CAD build for the part. Positions are in the model's coordinates, mm. A direction names the side the tool comes from. Give positions to 0.01 mm unless a question says otherwise; leave off trailing zeros. Write each loop counter-clockwise with the first axis right and the second up, starting at its lowest first coordinate (ties: lowest second). Pieces come first, ordered by that corner, then holes. Notation, with made-up numbers: (-21.5, 17.5) - (-7.5, 17.5) arc R24 cw to (-7.5, 34.5) - close; hole circle Ø6 at (1.25, 85). An arc over 180 degrees is marked (long way). Put each result on its own line as item: value. Start each with the question number.
1. Tool access for faces 1 (the cylindrical face through (-11.273, 178.043, -387.92)), 2 (the cylindrical face through (9.113, 196.684, -489.814)), 3 (the flat face through (-21, 47, 5)): list every direction of +Z, -Z, +X, -X, +Y, -Y with a clear straight run to the whole face (end or side of a thin tool).
2. Wall check: line 1 (Y direction, x = 30, z = -488); line 2 (Z direction, x = -25, y = 78); line 3 (X direction, y = -36, z = -171). Give the ranges that are in metal, low to high.
3. Cut at B-B on z = -130. List the corners of the cut face in (x, y).
4. Cut at C-C on x = -16.5. List the corners of the cut face in (y, z), and give its area (3 significant figures).
5. Cut at A-A on x = -44. List the corners of the cut face in (y, z).
6. Mould opens along X. For faces 4 (the flat face through (52, 122, -487.279)), 5 (the cylindrical face through (-49.95, 63.18, -246.29)), 6 (the cylindrical face through (-55.55, -42.594, 2.465)) say: +X half, -X half, draft (parallel to the pull), parting line (faces both ways), or undercut.
7. Drop flat-ended pins along their axis: pin 1 (5 mm diameter, centred on x = -11.5, y = 119.5, fed in from +Z); pin 2 (4.5 mm diameter, centred on x = 0, y = -60, fed in from +Z); pin 3 (4.5 mm diameter, centred on x = -30, y = 51.96, fed in from +Z); pin 4 (10 mm diameter, centred on x = 40, y = -33.5, fed in from -Z). Give the stop position or say it passes through.
from build123d import *

# Parameters (mm, degrees)
SKETCH2_R           = 52
SKETCH2_R_2         = 50
SKETCH4_R           = 70
SKETCH4_R_2         = 50
SKETCH4_R_3         = 2.5
BOSS_EXTRUDE1_DEPTH = 5
BOSS_EXTRUDE2_START = 5
SKETCH5_R           = 70
SKETCH5_R_2         = 50
SKETCH5_R_3         = 2.5
BOSS_EXTRUDE2_DEPTH = 5


with BuildPart() as part:
    # Sweep-Thin1: sweep along a path in Sketch3
    with BuildLine(Plane(origin=(0, 0, 0), x_dir=(0, 0, -1), z_dir=(1, 0, 0))) as sweep_thin1_path:
        Line((0, 0), (180, 0))
        Line((180, 0), (307.279220614, 127.279220614))
        Line((307.279220614, 127.279220614), (487.279220614, 127.279220614))
    # Sketch2 → Sweep-Thin1 (sweep)
    with BuildSketch(Plane.XY):
        Circle(SKETCH2_R)
        Circle(SKETCH2_R_2, mode=Mode.SUBTRACT)
    sweep(path=sweep_thin1_path.line, transition=Transition.RIGHT)

    # Sketch4 → Boss-Extrude1 (add)
    with BuildSketch(Plane.XY):
        Circle(SKETCH4_R)
        with Locations(Location((0, 0, 0), (0, 0, 90))):
            Circle(SKETCH4_R_2, mode=Mode.SUBTRACT)
        with Locations((0, -60)):
            Circle(SKETCH4_R_3, mode=Mode.SUBTRACT)
        with Locations((-30, -51.961524227)):
            Circle(SKETCH4_R_3, mode=Mode.SUBTRACT)
        with Locations((-51.961524227, -30)):
            Circle(SKETCH4_R_3, mode=Mode.SUBTRACT)
        with Locations((-60, 0)):
            Circle(SKETCH4_R_3, mode=Mode.SUBTRACT)
        with Locations((-51.961524227, 30)):
            Circle(SKETCH4_R_3, mode=Mode.SUBTRACT)
        with Locations((-30, 51.961524227)):
            Circle(SKETCH4_R_3, mode=Mode.SUBTRACT)
        with Locations((0, 60)):
            Circle(SKETCH4_R_3, mode=Mode.SUBTRACT)
        with Locations((30, 51.961524227)):
            Circle(SKETCH4_R_3, mode=Mode.SUBTRACT)
        with Locations((51.961524227, 30)):
            Circle(SKETCH4_R_3, mode=Mode.SUBTRACT)
        with Locations((60, 0)):
            Circle(SKETCH4_R_3, mode=Mode.SUBTRACT)
        with Locations((51.961524227, -30)):
            Circle(SKETCH4_R_3, mode=Mode.SUBTRACT)
        with Locations((30, -51.961524227)):
            Circle(SKETCH4_R_3, mode=Mode.SUBTRACT)
    extrude(amount=BOSS_EXTRUDE1_DEPTH)

    # Sketch5 → Boss-Extrude2 (add)
    with BuildSketch(Plane(origin=(0, 0, -487.279220614), x_dir=(-1, 0, 0), z_dir=(0, 0, -1)).offset(BOSS_EXTRUDE2_START)):
        with Locations((0, 127.279220614)):
            Circle(SKETCH5_R)
        with Locations((0, 127.279220614)):
            Circle(SKETCH5_R_2, mode=Mode.SUBTRACT)
        with Locations((0, 67.279220614)):
            Circle(SKETCH5_R_3, mode=Mode.SUBTRACT)
        with Locations((-30, 75.317696387)):
            Circle(SKETCH5_R_3, mode=Mode.SUBTRACT)
        with Locations((-51.961524227, 97.279220614)):
            Circle(SKETCH5_R_3, mode=Mode.SUBTRACT)
        with Locations((-60, 127.279220614)):
            Circle(SKETCH5_R_3, mode=Mode.SUBTRACT)
        with Locations((-51.961524227, 157.279220614)):
            Circle(SKETCH5_R_3, mode=Mode.SUBTRACT)
        with Locations((-30, 179.240744841)):
            Circle(SKETCH5_R_3, mode=Mode.SUBTRACT)
        with Locations((0, 187.279220614)):
            Circle(SKETCH5_R_3, mode=Mode.SUBTRACT)
        with Locations((30, 179.240744841)):
            Circle(SKETCH5_R_3, mode=Mode.SUBTRACT)
        with Locations((51.961524227, 157.279220614)):
            Circle(SKETCH5_R_3, mode=Mode.SUBTRACT)
        with Locations((60, 127.279220614)):
            Circle(SKETCH5_R_3, mode=Mode.SUBTRACT)
        with Locations((51.961524227, 97.279220614)):
            Circle(SKETCH5_R_3, mode=Mode.SUBTRACT)
        with Locations((30, 75.317696387)):
            Circle(SKETCH5_R_3, mode=Mode.SUBTRACT)
    extrude(amount=-BOSS_EXTRUDE2_DEPTH)


solid = part.part
Report:
1. face 1: none
1. face 2: -Z
1. face 3: +Z, +X, -X, +Y, -Y
2. line 1: y = 64.03 to 72.82, 77.82 to 87.28, 167.28 to 176.74, 181.74 to 190.52
2. line 2: z = -492.28 to -487.28, -322.48 to -319.24, -196.76 to -193.52
2. line 3: x = -37.52 to -34.7, 34.7 to 37.52
3. outline: circle Ø104 at (0, 0); hole circle Ø100 at (0, 0)
4. outline: (-68.03, 0) - (-49.31, 0) - (-49.31, -200.43) - (77.97, -327.71) - (77.97, -487.28) - (59.25, -487.28) - (59.25, -492.28) - (80.08, -492.28) - (80.08, -326.83) - (-47.2, -199.55) - (-47.2, 5) - (-68.03, 5) - close; (47.2, -160.45) - (174.48, -287.73) - (174.48, -492.28) - (195.31, -492.28) - (195.31, -487.28) - (176.59, -487.28) - (176.59, -286.85) - (49.31, -159.57) - (49.31, 0) - (68.03, 0) - (68.03, 5) - (47.2, 5) - close
4. area: 2,700 mm²
5. outline: (-54.44, 0) - (-27.71, 0) - (-27.71, -191.48) - (99.57, -318.76) - (99.57, -487.28) - (72.84, -487.28) - (72.84, -492.28) - (103.53, -492.28) - (103.53, -317.12) - (-23.75, -189.84) - (-23.75, 5) - (-54.44, 5) - close; (23.75, -170.16) - (151.03, -297.44) - (151.03, -492.28) - (181.72, -492.28) - (181.72, -487.28) - (154.99, -487.28) - (154.99, -295.8) - (27.71, -168.52) - (27.71, 0) - (54.44, 0) - (54.44, 5) - (23.75, 5) - close
6. face 4: draft
6. face 5: undercut
6. face 6: parting line
7. pin 1: stops at z = -225.16
7. pin 2: passes through
7. pin 3: stops at z = -168.77
7. pin 4: stops at z = -202.57
